Geometry: final body of the model. Coordinates: model frame, mm. Give positions to 0.01 mm unless a question says otherwise; leave off trailing zeros. Write each loop counter-clockwise with the first axis right and the second up, starting at its lowest first coordinate (ties: lowest second). Pieces come first, ordered by that corner, then holes. Notation, with made-up numbers: (-22, -32) -> (-9, -32) arc R18 cw to (-9, -15) -> close; hole circle Ø11 at (60.5, 73). An arc over 180 degrees is marked (long way). Answer as a JSON object with one key per item and string values. Group by question number.
(1) Draft query along Z for faces 1 (the face through (-20.438, -14.155, -6.436)), 2 (the face through (2.25, 7.13, 10.15)). Return one class per face: +Z half, -Z half, draft (parallel to the pull), parting line (faces both ways), or undercut.
(2) Section query D-D on y = -7. Output: boundary loops of the cut face in (x, z).
(3) Section query A-A on z = 0. Output: boundary loops of the cut face in (x, y).
(4) Material intervals for probe 1 along Y at (x, z) = (6, 9); probe 2 along Y at (x, z) = (-9, 5.5); probe 3 along X at (y, z) = (-35.5, 6), sorted ascending.
(5) Section query B-B on y = -18. Output: boundary loops of the cut face in (x, z).
(6) Contact query for flat-ended pins moving along their axis: pin 1 Ø12 at (y, z) = (4, -5) entering from +X; pin 2 Ø3 at (x, y) = (16.5, -29.5) entering from -Z; pin 3 Ø8 at (x, y) = (-11, 1.5) entering from -Z. Output: stop coordinate, or through.
(7) Section query C-C on x = 0. Output: boundary loops of the cut face in (y, z).
from build123d import *


with BuildPart() as f1:
    # F0 (on Top) → F1 (revolve)
    with BuildSketch(Plane.XY):
        with BuildLine():
            ThreePointArc((0, -13.5107505449), (-11.3620086767, -6.4847930924), (-10.1525229381, 6.8192086943))
            ThreePointArc((-10.1525229381, 6.8192086943), (-15.9881985309, -2.5605712732), (-14.5291043663, -13.5107505449))
            Line((-14.5291043663, -13.5107505449), (0, -13.5107505449))
        make_face()
        with BuildLine():
            ThreePointArc((-14.5291043663, -13.5107505449), (-15.9881985309, -2.5605712732), (-10.1525229381, 6.8192086943))
            Line((-10.1525229381, 6.8192086943), (-14.0944705725, 11.7975165241))
            ThreePointArc((-14.0944705725, 11.7975165241), (-21.8076146048, 0.3158808225), (-21.4270698922, -13.5107505449))
            Line((-21.4270698922, -13.5107505449), (-14.5291043663, -13.5107505449))
        make_face()
        Polygon((0, -14.7807505449), (0, -13.5107505449), (-14.5291043663, -13.5107505449), (-21.4270698922, -13.5107505449), (-21.4270698922, -14.7807505449), (-14.5291043663, -14.7807505449), align=None)
        with BuildLine():
            ThreePointArc((-10.1525229381, -35.110709784), (-11.3620086767, -21.8067079973), (0, -14.7807505449))
            Line((0, -14.7807505449), (-14.5291043663, -14.7807505449))
            ThreePointArc((-14.5291043663, -14.7807505449), (-15.9881985309, -25.7309298165), (-10.1525229381, -35.110709784))
        make_face()
        with BuildLine():
            ThreePointArc((-10.1525229381, -35.110709784), (-15.9881985309, -25.7309298165), (-14.5291043663, -14.7807505449))
            Line((-14.5291043663, -14.7807505449), (-21.4270698922, -14.7807505449))
            ThreePointArc((-21.4270698922, -14.7807505449), (-21.8076146048, -28.6073819122), (-14.0944705725, -40.0890176138))
            Line((-14.0944705725, -40.0890176138), (-10.1525229381, -35.110709784))
        make_face()
    revolve(axis=Axis((0, -14.1457505449, 0), (0, -1, 0)))


solid = f1.part
Answer list:
{
 "1": {"face 1": "parting line", "face 2": "undercut"},
 "2": {"outline": "circle Ø45.37 at (0, 0); hole circle Ø22.18 at (0, 0)"},
 "3": {"outline": "(-21.43, -14.78) arc R22.7 ccw to (-14.09, -40.09) -> (-10.15, -35.11) arc R12.7 cw (long way) to (10.15, -35.11) -> (14.09, -40.09) arc R22.7 ccw to (21.43, -14.78) -> (21.43, -13.51) arc R22.7 ccw to (14.09, 11.8) -> (10.15, 6.82) arc R12.7 cw (long way) to (-10.15, 6.82) -> (-14.09, 11.8) arc R22.7 ccw to (-21.43, -13.51) -> close"},
 "4": {"probe 1": "-35.95 to -34.14, -20.83 to -7.47, 5.84 to 7.66", "probe 2": "-35.61 to -34.55, -20.41 to -7.88, 6.26 to 7.32", "probe 3": "-17.46 to -8.57, 8.57 to 17.46"},
 "5": {"outline": "circle Ø44.59 at (0, 0); hole circle Ø16.9 at (0, 0)"},
 "6": {"pin 1": "x = 22.11", "pin 2": "z = -15.59", "pin 3": "z = -20.71"},
 "7": {"outline": "(-40.09, -14.09) arc R22.7 ccw to (-14.78, -21.43) -> (-13.51, -21.43) arc R22.7 ccw to (11.8, -14.09) -> (6.82, -10.15) arc R12.7 cw (long way) to (6.82, 10.15) -> (11.8, 14.09) arc R22.7 ccw to (-13.51, 21.43) -> (-14.78, 21.43) arc R22.7 ccw to (-40.09, 14.09) -> (-35.11, 10.15) arc R12.7 cw (long way) to (-35.11, -10.15) -> close"}
}
